```python
from build123d import *

# Parameters (mm, degrees)
F0_R      = 45
F1_DEPTH  = 10
F2_R      = 24.5
F2_R_2    = 20
F3_DEPTH  = 140
F4_R      = 20
F5_DEPTH  = 150.001
F6_R      = 45
F6_R_2    = 20
F7_DEPTH  = 10
F8_R      = 4.25
F9_DEPTH  = 160.001
F12_R     = 18.5
F13_DEPTH = 90
F14_R     = 28.5
F15_DEPTH = 10
F16_R     = 14
F17_DEPTH = 90
F18_R     = 2.25
F19_DEPTH = 12


with BuildPart() as f1:
    # F0 (on Top) → F1 (new body)
    with BuildSketch(Plane.XY):
        Circle(F0_R)
    extrude(amount=F1_DEPTH)

    # F2 (on face) → F3 (join)
    with BuildSketch(Plane.XY.offset(10)):
        Circle(F2_R)
        Circle(F2_R_2, mode=Mode.SUBTRACT)
    extrude(amount=F3_DEPTH)

    # F4 (on face) → F5 (cut, through all)
    with BuildSketch(Plane(origin=(0, 0, 0), x_dir=(1, 0, 0), z_dir=(0, 0, -1))):
        Circle(F4_R)
    extrude(amount=-F5_DEPTH, mode=Mode.SUBTRACT)

    # F6 (on face) → F7 (join)
    with BuildSketch(Plane.XY.offset(150)):
        Circle(F6_R)
        Circle(F6_R_2, mode=Mode.SUBTRACT)
    extrude(amount=F7_DEPTH)

    # F8 (on face) → F9 (cut, through all)
    with BuildSketch(Plane.XY.offset(160)):
        with Locations((0, 35)):
            Circle(F8_R)
        with Locations((0, -35)):
            Circle(F8_R)
        with Locations((35, 0)):
            Circle(F8_R)
        with Locations((-35, 0)):
            Circle(F8_R)
        with Locations((-24.733197, 24.764268)):
            Circle(F8_R)
        with Locations((24.733197, -24.764268)):
            Circle(F8_R)
        with Locations((-24.827064, -24.670162)):
            Circle(F8_R)
        with Locations((24.638896, 24.858094)):
            Circle(F8_R)
    extrude(amount=-F9_DEPTH, mode=Mode.SUBTRACT)

    # F12 (on face) → F13 (join)
    with BuildSketch(Plane(origin=(-82.744423, 0, 85.045383), x_dir=(0.716736, 0, 0.697344), z_dir=(-0.697344, 0, 0.716736))):
        with Locations((28.086591, 0)):
            Circle(F12_R)
    extrude(amount=-F13_DEPTH)

    # F14 (on face) → F15 (join)
    with BuildSketch(Plane(origin=(-82.744423, 0, 85.045383), x_dir=(0.716736, 0, 0.697344), z_dir=(-0.697344, 0, 0.716736))):
        with Locations((28.086591, 0)):
            Circle(F14_R)
    extrude(amount=-F15_DEPTH)

    # F16 (on face) → F17 (cut)
    with BuildSketch(Plane(origin=(-82.744423, 0, 85.045383), x_dir=(0.716736, 0, 0.697344), z_dir=(-0.697344, 0, 0.716736))):
        with Locations((28.086591, 0)):
            Circle(F16_R)
    extrude(amount=-F17_DEPTH, mode=Mode.SUBTRACT)

    # F18 (on face) → F19 (cut)
    with BuildSketch(Plane(origin=(-82.744423, 0, 85.045383), x_dir=(0.716736, 0, 0.697344), z_dir=(-0.697344, 0, 0.716736))):
        with Locations((26.669547, 21.451613)):
            Circle(F18_R)
        with Locations((6.909627, 0)):
            Circle(F18_R)
        with Locations((26.669547, -21.075269)):
            Circle(F18_R)
        with Locations((49.064126, 0)):
            Circle(F18_R)
    extrude(amount=-F19_DEPTH, mode=Mode.SUBTRACT)


solid = f1.part
```
The model under review builds one solid part; all positions refer to its coordinate system, in mm. A direction names the side the tool comes from. Round coordinates to 2 decimals unless told otherwise and drop trailing zeros. Order: outer loops, then holes, each group sorted by start corner. A loop starts at its lowest first (then second) coordinate and runs counter-clockwise, first axis right, second up. Notation, with made-up numbers: (87, 15) -> (93, 15) arc R29 cw to (93, 49) -> close; hole circle Ø10 at (36.25, -29.75). An arc over 180 degrees is marked (long way). Use a Markdown table: item, result.
Q1. Tool access review of faces 1 (the flat face through (19, -19, 150)), 2 (the flat face through (-9.737, 4.197, 30.509)), 3 (the cylindrical face through (-39.246, 0.187, 155.07)), 4 (the cylindrical face through (21.506, 27.73, 155.07)): name each direction out of +Z, -Z, +X, -X, +Y, -Y from which nothing blocks a thin tool from reaching the whole face with its end or side.
Values:
| item | result |
|---|---|
| face 1 | none |
| face 2 | -Z |
| face 3 | +Z |
| face 4 | +Z, -Z |
Q2. We need section A-A on x = 16. Write out the cut boundary in (y, z), then the cut area to 3 significant figures.
Values:
| item | result |
|---|---|
| outline | (-42.06, 0) -> (-12, 0) -> (-12, 160) -> (-42.06, 160) -> (-42.06, 150) -> (-18.55, 150) -> (-18.55, 10) -> (-42.06, 10) -> close; (12, 0) -> (42.06, 0) -> (42.06, 10) -> (18.55, 10) -> (18.55, 150) -> (42.06, 150) -> (42.06, 160) -> (12, 160) -> close |
| area | 3,040 mm^2 |
Q3. Mouldability with a two-part tool opening along Y and no side actions: class faces 5 (the flat face through (19, -19, 10)), 6 (the cylindrical face through (-25.38, -20.456, 5.07)), 7 (the cylindrical face through (-51.916, 0.813, 67.132)) as +Y half, -Y half, draft (parallel to the pull), parting line (faces both ways), or undercut.
Values:
| item | result |
|---|---|
| face 5 | draft |
| face 6 | undercut |
| face 7 | parting line |
Q4. Clearance check with flat-ended pins moving along their axes: P1, Ø10, axis at x = 24.73, y = -24.76, coming from the +Z side; P2, Ø5, axis at y = -14, z = 73.5, coming from the -X side; P3, Ø7.5, axis at x = 0, y = -35, coming from the -Z side; P4, Ø8, axis at y = -20, z = 117.5, coming from the +X side. State where each tip first meets the part, or that it passes through.
Values:
| item | result |
|---|---|
| P1 | stops at z = 160 |
| P2 | stops at x = -53.43 |
| P3 | passes through |
| P4 | stops at x = 18.55 |
Q5. We need section D-D on y = 0. State how many separate pieces and enclosed holes the cut face has, then the cut area to 3 significant figures.
Values:
| item | result |
|---|---|
| separate pieces | 9 |
| enclosed holes | 0 |
| area | 2,600 mm^2 |
Q6. We need section C-C on z = 19.5. Write out the cut boundary in (x, y).
Values:
| item | result |
|---|---|
| outline | circle Ø49 at (0, 0); hole circle Ø40 at (0, 0) |
Q7. We need section B-B on y = 35. Write out the cut boundary in (x, z).
Values:
| item | result |
|---|---|
| outline | (-28.28, 0) -> (-4.25, 0) -> (-4.25, 10) -> (-28.28, 10) -> close; (-28.28, 150) -> (-4.25, 150) -> (-4.25, 160) -> (-28.28, 160) -> close; (4.25, 0) -> (28.28, 0) -> (28.28, 10) -> (4.25, 10) -> close; (4.25, 150) -> (28.28, 150) -> (28.28, 160) -> (4.25, 160) -> close |
Q8. For line 1 (Y direction, x = 0, z = 152.5); line 2 (X direction, y = -3, z = 61.5); line 3 (Y direction, x = 0, z = 32), list the stretches that pass through material, from the lowest coordinate up.
Values:
| item | result |
|---|---|
| line 1 | y = -45 to -39.25, -30.75 to -20, 20 to 30.75, 39.25 to 45 |
| line 2 | x = -46.12 to -39.73, -1.57 to 4.82, 19.77 to 24.32 |
| line 3 | y = -24.5 to -20, 20 to 24.5 |
